For this review, use the dimensioned drawing (mm, ordinates from the lowest corner) and the shaded views. A direction names the side the tool comes from. Coordinates: 2 decimals unless noted, no trailing zeros. Loops run counter-clockwise (first coordinate to the right, second up) from the corner with the lowest first, then second, coordinate; pieces in that order, holes last. Notation, with made-up numbers: (-15.75, 67) - (3.25, 67) arc R29 cw to (3.25, 96) - close; hole circle Ø5 at (-21, 34). An arc over 180 degrees is marked (long way). Use a Markdown table: item, result. Add a question column.
1) Add section C-C, the plane y = 5.25. Give the boundary of the cut face in (x, z), and give its area (3 significant figures).
2) For the marked faces 4 and 5, list the 3-axis set-ups (+Z, -Z, +X, -X, +Y, -Y) from which the entire face can be reached by the end or side of a thin tool; tool diameter is ignored.
3) The part is to be moulded in two halves that separate along X. For the marked faces 1, 2 and 3, say which applies: pulls with the +X half, pulls with the -X half, needs draft (parallel to the pull), parting line crosses it, or undercut.
4) To check wall thickness, follow L1, parallel to Z at x = 4.4, y = 5.25; L2, parallel to Y at x = 0.75, z = 6.25; L3, parallel to Y at x = 1.5, z = 6.5. State the ranges of each line that lie inside material, in increasing order. Write a range as [from, to].
5) Clearance check with flat-ended pins moving along their axes: pin 1 (1 mm diameter, centred on x = 1, y = 2, fed in from +Z); pin 2 (1.5 mm diameter, centred on x = 1.5, z = 1, fed in from -Y). State where each tip first meets the part, or that it passes through.
6) Add section A-A, the plane x = 4.4. Give the boundary of the cut face in (y, z), and give its area (3 significant figures).
7) Add section B-B, the plane y = 6.5. Give the boundary of the cut face in (x, z).
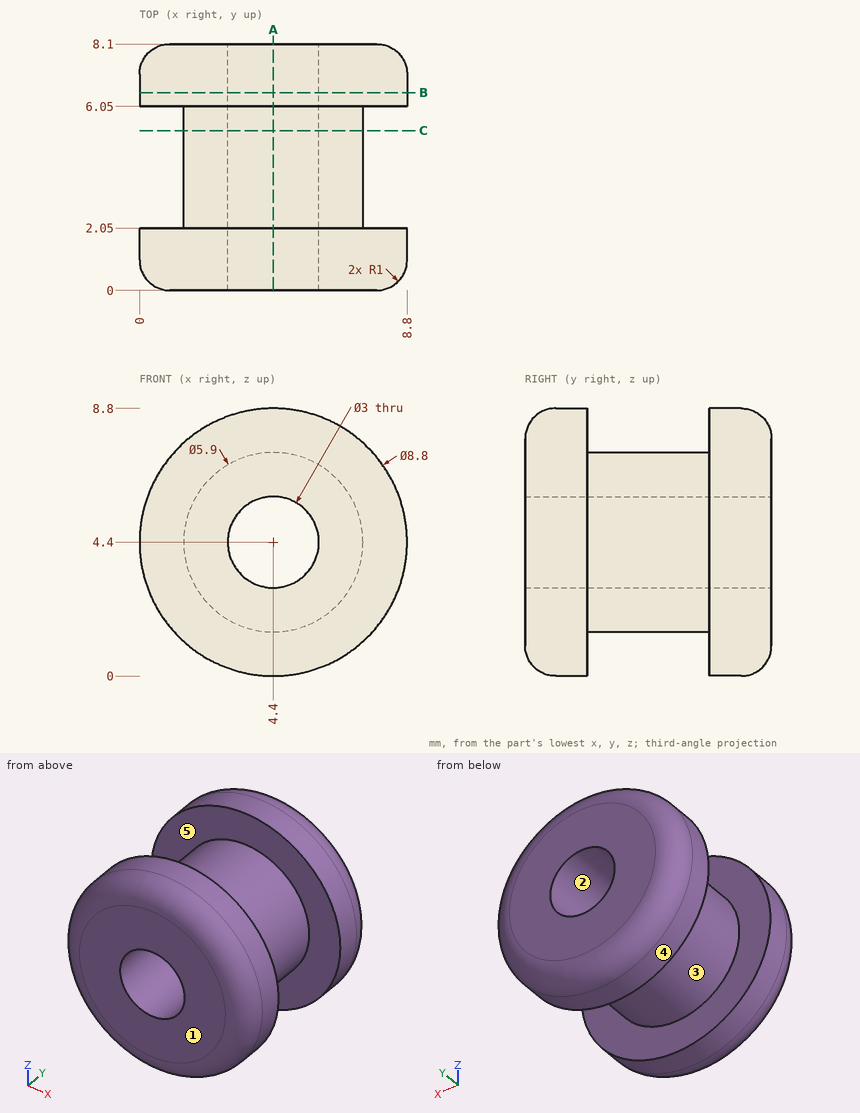
From the geometry:
| question | item | result |
|---|---|---|
| 1 | outline | circle Ø5.9 at (4.4, 4.4); hole circle Ø3 at (4.4, 4.4) |
| 1 | area | 20.3 mm^2 |
| 2 | face 4 | +Y, -Y |
| 2 | face 5 | none |
| 3 | face 1 | needs draft |
| 3 | face 2 | undercut |
| 3 | face 3 | parting line crosses it |
| 4 | L1 | z = [1.45, 2.9], [5.9, 7.35] |
| 4 | L2 | y = [0.28, 2.05], [6.05, 7.82] |
| 4 | L3 | y = [0.02, 2.05], [6.05, 8.08] |
| 5 | pin 1 | stops at z = 7.71 |
| 5 | pin 2 | stops at y = 0.05 |
| 6 | outline | (0, 1) arc R1 ccw to (1, 0) - (2.05, 0) - (2.05, 1.45) - (6.05, 1.45) - (6.05, 0) - (7.1, 0) arc R1 ccw to (8.1, 1) - (8.1, 2.9) - (0, 2.9) - close; (0, 5.9) - (8.1, 5.9) - (8.1, 7.8) arc R1 ccw to (7.1, 8.8) - (6.05, 8.8) - (6.05, 7.35) - (2.05, 7.35) - (2.05, 8.8) - (1, 8.8) arc R1 ccw to (0, 7.8) - close |
| 6 | area | 34.5 mm^2 |
| 7 | outline | circle Ø8.8 at (4.4, 4.4); hole circle Ø3 at (4.4, 4.4) |
